The model under review builds one solid part; all positions refer to its coordinate system, in mm. A direction names the side the tool comes from. Give positions to 0.01 mm unless a question says otherwise; leave off trailing zeros. Order: outer loops, then holes, each group sorted by start corner. A loop starts at its lowest first (then second) coordinate and runs counter-clockwise, first axis right, second up. Notation, with made-up numbers: (-8, 57.5) - (50, 57.5) arc R30 ccw to (50, 94.5) - close; hole circle Ø3 at (50.25, 34). An arc over 180 degrees is marked (long way). Write item = value, one per line. Start each with the question number.
1. Mouldability with a two-part tool opening along X and no side actions: class faces 1 (the flat face through (38.1, 28, -9)), 2 (the flat face through (0, 19, -9)), 3 (the flat face through (57.15, 19, -9)) as pulls with the +X half, pulls with the -X half, needs draft (parallel to the pull), parting line crosses it, or undercut.
2. Machinability: for faces 4 (the flat face through (28, 15, 0)), 5 (the flat face through (19.05, 29, -9)), which of the approach directions +Z, -Z, +X, -X, +Y, -Y give a long, thin tool a straight path to every point of the face, cutting with its end or side? Answer none if there is none.
3. We need section A-A, the plane y = 34. Give the boundary of the cut face in (x, z), and give its area (3 significant figures).
4. Wall thickness on probe 1 along X at (y, z) = (22, -4); probe 2 along Y at (x, z) = (24, -16): over which ranges is each line inside the solid? List them lowest first.
5. For P1, Ø1, axis at x = 29.5, z = -7.5, coming from the -Y side; P2, Ø3, axis at x = 26, z = -7.5, coming from the +Y side, all flat-tipped, find the tip position at first contact; note any pin that passes through.
6. We need section B-B, the plane z = -9. Give the boundary of the cut face in (x, y), and give its area (3 significant figures).
7. We need section C-C, the plane x = 36. Give the boundary of the cut face in (y, z), and give its area (3 significant figures).
Autodesk Inventor part; units mm, degrees
ref_plane "YZ Plane" through (0, 0, 0) normal (1, 0, 0) x (0, 1, 0)
ref_plane "XZ Plane" through (0, 0, 0) normal (0, 1, 0) x (-1, 0, 0)
ref_plane "XY Plane" through (0, 0, 0) normal (0, 0, 1) x (1, 0, 0)
sketch "Sketch1" plane through (0, 0, 0) normal (0, 0, 1) x (1, 0, 0)
  point P0 (0, 0)
sketch "Sketch2" plane through (0, 0, 0) normal (0, 0, 1) x (1, 0, 0)
  line L0 (0, 38.1) -> (0, 0)
  line L1 (0, 38.1) -> (19.05, 38.1)
  line L2 (19.05, 38.1) -> (19.05, 19.05)
  line L3 (19.05, 19.05) -> (38.1, 19.05)
  line L4 (38.1, 19.05) -> (38.1, 38.1)
  line L5 (38.1, 38.1) -> (57.15, 38.1)
  line L6 (57.15, 38.1) -> (57.15, 0)
  line L7 (57.15, 0) -> (0, 0)
  dimension "d0" = 38.1
  dimension "d1" = 19.05
  dimension "d2" = 19.05
  dimension "d3" = 19.05
  dimension "d4" = 19.05
  dimension "d5" = 19.05
extrude "Extrusion1" add sketch "Sketch2" against normal blind 19.05
equation "\"d0\" = 2 * cube"
equation "\"d1\" = cube"
equation "\"d2\" = cube"
equation "\"d3\" = cube"
equation "\"d5\" = cube"
equation "\"d6\" = cube"
equation "\"cube\" = 19.05"
properties part number "IED7_Sun_PuzzleCubeRed"
Model answer:
q1.face_1 = undercut
q1.face_2 = pulls with the -X half
q1.face_3 = pulls with the +X half
q2.face_4 = +Z, +X, -X, +Y, -Y
q2.face_5 = +Z, -Z, +Y
q3.outline = (0, -19.05) - (19.05, -19.05) - (19.05, 0) - (0, 0) - close; (38.1, -19.05) - (57.15, -19.05) - (57.15, 0) - (38.1, 0) - close
q3.area = 726 mm2
q4.probe_1 = 0 to 19.05, 38.1 to 57.15
q4.probe_2 = 0 to 19.05
q5.P1 = 0
q5.P2 = 19.05
q6.outline = (0, 0) - (57.15, 0) - (57.15, 38.1) - (38.1, 38.1) - (38.1, 19.05) - (19.05, 19.05) - (19.05, 38.1) - (0, 38.1) - close
q6.area = 1,810 mm2
q7.outline = (0, -19.05) - (19.05, -19.05) - (19.05, 0) - (0, 0) - close
q7.area = 363 mm2
